Design review of the part built by this model. Coordinates are the model's own, in mm. A direction names the side the tool comes from. Coordinates: 2 decimals unless noted, no trailing zeros. Write each loop counter-clockwise with the first axis right and the second up, starting at its lowest first coordinate (ties: lowest second). Pieces come first, ordered by that corner, then holes.
Q1. Clearance check with flat-ended pins moving along their axes: pin 1 Ø4 at (x, y) = (16, 34) entering from -Z; pin 2 Ø1 at (x, y) = (30.5, -14.5) entering from +Z; pin 3 Ø6 at (x, z) = (54.5, 13.5) entering from -Y. State where each tip first meets the part, or that it passes through.
Q2. To check wall thickness, follow probe 1 along Z at (x, y) = (15, 9); probe 2 along Z at (x, y) = (122.5, 73.5). State the ranges of each line that lie inside material, in increasing order.
Q3. Add section C-C, the plane x = 16.5. Give the boundary of the cut face in (y, z).
Q4. Add section A-A, the plane y = 9. Give the boundary of the cut face in (x, z).
Q5. Machinability: for faces 1 (the face through (38, -96.838, -1)), 2 (the face through (38, 96.838, -1)), 3 (the face through (38, 1, -96.838)), which of the approach directions +Z, -Z, +X, -X, +Y, -Y give a long, thin tool a straight path to every point of the face, cutting with its end or side? Answer none if there is none.
from build123d import *

# Parameters (mm, degrees)
F0_W     = 203.2
F0_H     = 203.2
F1_DEPTH = 127
F2_W     = 203.2
F2_H     = 203.2
F2_W_2   = 193.675
F2_H_2   = 193.675
F3_DEPTH = 76.2
F4_R     = 5.08


with BuildPart() as f1:
    # F0 (on Right) → F1 (new body)
    with BuildSketch(Plane.YZ):
        Rectangle(F0_W, F0_H)
    extrude(amount=F1_DEPTH)

    # F2 (on face) → F3 (cut)
    with BuildSketch(Plane(origin=(0, 0, 0), x_dir=(0, -1, 0), z_dir=(-1, 0, 0))):
        Rectangle(F2_W, F2_H)
        Rectangle(F2_W_2, F2_H_2, mode=Mode.SUBTRACT)
    extrude(amount=-F3_DEPTH, mode=Mode.SUBTRACT)

    # F4
    f4_edges = [f1.edges().sort_by_distance(p)[0] for p in [
        (101.6, 101.6, 101.6),
        (127, 101.6, 0),
        (101.6, 101.6, -101.6),
        (127, 0, -101.6),
        (127, 0, 101.6),
        (127, -101.6, 0),
        (101.6, -101.6, 101.6),
        (101.6, -101.6, -101.6),
    ]]
    fillet(f4_edges, radius=F4_R)


solid = f1.part
Here are the results:
1. pin 1: stops at z = -96.84
1. pin 2: stops at z = 96.84
1. pin 3: stops at y = -96.84
2. probe 1: z = -96.84 to 96.84
2. probe 2: z = -101.57 to 101.57
3. outline: (-96.84, -96.84) - (96.84, -96.84) - (96.84, 96.84) - (-96.84, 96.84) - close
4. outline: (0, -96.84) - (76.2, -96.84) - (76.2, -101.6) - (121.92, -101.6) arc R5.08 ccw to (127, -96.52) - (127, 96.52) arc R5.08 ccw to (121.92, 101.6) - (76.2, 101.6) - (76.2, 96.84) - (0, 96.84) - close
5. face 1: +Z, -Z, -X, -Y
5. face 2: +Z, -Z, -X, +Y
5. face 3: -Z, -X, +Y, -Y
